```python
from build123d import *

# Parameters (mm, degrees)
SKETCH003_W                  = 82
SKETCH003_H                  = 82
PAD002_DEPTH                 = 3
SKETCH004_R                  = 3.5
POCKET_DEPTH                 = 3
SKETCH004_LINEARPATTERN_2_R  = 3.5
POCKET_LINEARPATTERN_2_DEPTH = 3
SKETCH004_LINEARPATTERN_3_R  = 3.5
POCKET_LINEARPATTERN_3_DEPTH = 3
SKETCH004_LINEARPATTERN_4_R  = 3.5
POCKET_LINEARPATTERN_4_DEPTH = 3
SKETCH004_LINEARPATTERN_5_R  = 3.5
POCKET_LINEARPATTERN_5_DEPTH = 3
SKETCH004_LINEARPATTERN_6_R  = 3.5
POCKET_LINEARPATTERN_6_DEPTH = 3
SKETCH004_LINEARPATTERN_7_R  = 3.5
POCKET_LINEARPATTERN_7_DEPTH = 3
SKETCH004_LINEARPATTERN_8_R  = 3.5
POCKET_LINEARPATTERN_8_DEPTH = 3
LINEARPATTERN001_COUNT       = 8
LINEARPATTERN001_PITCH       = 10


with BuildPart() as part:
    # Sketch003 → Pad002 (new body)
    with BuildSketch(Plane.XZ):
        Rectangle(SKETCH003_W, SKETCH003_H)
    extrude(amount=-PAD002_DEPTH)

    # Sketch004 → Pocket (cut)
    with BuildSketch(Plane.XZ):
        with Locations((-35, 34.963)):
            Circle(SKETCH004_R)
    pocket = extrude(amount=-POCKET_DEPTH, mode=Mode.SUBTRACT)

    # Sketch004 LinearPattern 2 → Pocket LinearPattern 2 (cut)
    with BuildSketch(Plane(origin=(10, 0, 0), x_dir=(1, 0, 0), z_dir=(0, -1, 0))):
        with Locations((-35, 34.963)):
            Circle(SKETCH004_LINEARPATTERN_2_R)
    pocket_linearpattern_2 = extrude(amount=-POCKET_LINEARPATTERN_2_DEPTH, mode=Mode.SUBTRACT)

    # Sketch004 LinearPattern 3 → Pocket LinearPattern 3 (cut)
    with BuildSketch(Plane(origin=(20, 0, 0), x_dir=(1, 0, 0), z_dir=(0, -1, 0))):
        with Locations((-35, 34.963)):
            Circle(SKETCH004_LINEARPATTERN_3_R)
    pocket_linearpattern_3 = extrude(amount=-POCKET_LINEARPATTERN_3_DEPTH, mode=Mode.SUBTRACT)

    # Sketch004 LinearPattern 4 → Pocket LinearPattern 4 (cut)
    with BuildSketch(Plane(origin=(30, 0, 0), x_dir=(1, 0, 0), z_dir=(0, -1, 0))):
        with Locations((-35, 34.963)):
            Circle(SKETCH004_LINEARPATTERN_4_R)
    pocket_linearpattern_4 = extrude(amount=-POCKET_LINEARPATTERN_4_DEPTH, mode=Mode.SUBTRACT)

    # Sketch004 LinearPattern 5 → Pocket LinearPattern 5 (cut)
    with BuildSketch(Plane(origin=(40, 0, 0), x_dir=(1, 0, 0), z_dir=(0, -1, 0))):
        with Locations((-35, 34.963)):
            Circle(SKETCH004_LINEARPATTERN_5_R)
    pocket_linearpattern_5 = extrude(amount=-POCKET_LINEARPATTERN_5_DEPTH, mode=Mode.SUBTRACT)

    # Sketch004 LinearPattern 6 → Pocket LinearPattern 6 (cut)
    with BuildSketch(Plane(origin=(50, 0, 0), x_dir=(1, 0, 0), z_dir=(0, -1, 0))):
        with Locations((-35, 34.963)):
            Circle(SKETCH004_LINEARPATTERN_6_R)
    pocket_linearpattern_6 = extrude(amount=-POCKET_LINEARPATTERN_6_DEPTH, mode=Mode.SUBTRACT)

    # Sketch004 LinearPattern 7 → Pocket LinearPattern 7 (cut)
    with BuildSketch(Plane(origin=(60, 0, 0), x_dir=(1, 0, 0), z_dir=(0, -1, 0))):
        with Locations((-35, 34.963)):
            Circle(SKETCH004_LINEARPATTERN_7_R)
    pocket_linearpattern_7 = extrude(amount=-POCKET_LINEARPATTERN_7_DEPTH, mode=Mode.SUBTRACT)

    # Sketch004 LinearPattern 8 → Pocket LinearPattern 8 (cut)
    with BuildSketch(Plane(origin=(70, 0, 0), x_dir=(1, 0, 0), z_dir=(0, -1, 0))):
        with Locations((-35, 34.963)):
            Circle(SKETCH004_LINEARPATTERN_8_R)
    pocket_linearpattern_8 = extrude(amount=-POCKET_LINEARPATTERN_8_DEPTH, mode=Mode.SUBTRACT)

    # LinearPattern001: Pocket, Pocket LinearPattern 2, Pocket LinearPattern 3, Pocket LinearPattern 4, Pocket LinearPattern 5, Pocket LinearPattern 6, Pocket LinearPattern 7, Pocket LinearPattern 8 ×8
    with Locations(*[(0, 0, -i * LINEARPATTERN001_PITCH) for i in range(1, LINEARPATTERN001_COUNT)]):
        add(pocket, mode=Mode.SUBTRACT)
        add(pocket_linearpattern_2, mode=Mode.SUBTRACT)
        add(pocket_linearpattern_3, mode=Mode.SUBTRACT)
        add(pocket_linearpattern_4, mode=Mode.SUBTRACT)
        add(pocket_linearpattern_5, mode=Mode.SUBTRACT)
        add(pocket_linearpattern_6, mode=Mode.SUBTRACT)
        add(pocket_linearpattern_7, mode=Mode.SUBTRACT)
        add(pocket_linearpattern_8, mode=Mode.SUBTRACT)


solid = part.part
```
The listing builds one solid part. Answer for the finished solid, in the listing's coordinates (mm). Round coordinates to 2 decimals unless told otherwise and drop trailing zeros. Return JSON: item names as keys, results as strings. Group by question number.
1. The part is cut by section A-A on x = 35. State how many separate pieces and enclosed holes the cut face has, then the cut area to 3 significant figures.
2. This flat-tipped pin is pushed along its axis until it touches: P1, Ø9, axis at x = -35, z = -15.037, coming from the -Y side. Where does it stop, or does it pass through?
3. The mould has two halves that part along Z. Classify faces 1 (the cylindrical face through (32.223, 1.479, -17.167)), 2 (the cylindrical face through (18.34, 1.48, -3.99)), 3 (the flat face through (-1, 3, 1)): pulls with the +Z half, pulls with the -Z half, needs draft (parallel to the pull), parting line crosses it, or undercut.
Resolved:
{
 "1": {"separate pieces": "9", "enclosed holes": "0", "area": "78.0 mm²"},
 "2": {"P1": "stops at y = 0"},
 "3": {"face 1": "undercut", "face 2": "undercut", "face 3": "needs draft"}
}
